Can you work these out from the model? Positions are in its coordinate system, mm. A direction names the side the tool comes from. Give positions to 0.01 mm unless a question says otherwise; leave off trailing zeros. Write each loop counter-clockwise with the first axis right and the second up, starting at its lowest first coordinate (ties: lowest second). Pieces come first, ordered by that corner, then holes. Notation, with made-up numbers: M 41,25 L 59,25 A7 cw 59,35 Z; hole C 74.5,14.5 d7. An arc over 180 degrees is marked long. Write each question's results on one line, items separated by ' | '.
from build123d import *

# Parameters (mm, degrees)
F0_R     = 1.190625
F1_DEPTH = 4.7625
F2_R     = 1.27


# Not quite as in the source:
# - a feature names something its author has since deleted; it is built from what else it names


with BuildPart() as f1:
    # F0 (on Front) → F1 (new body)
    with BuildSketch(Plane.XZ):
        with BuildLine():
            Line((0, 5.08), (5.08, 5.08))
            Line((5.08, 5.08), (5.08, 14.605))
            Line((5.08, 14.605), (5.08, 24.13))
            Line((5.08, 24.13), (0, 24.13))
            Line((0, 24.13), (0, 21.844))
            ThreePointArc((0, 21.844), (1.9756563466, 21.0256563466), (2.794, 19.05))
            ThreePointArc((2.794, 19.05), (1.9756563466, 17.0743436534), (0, 16.256))
            Line((0, 16.256), (0, 5.08))
        make_face()
        with BuildLine():
            Line((-5.08, 5.08), (0, 5.08))
            Line((0, 5.08), (0, 16.256))
            ThreePointArc((0, 16.256), (-2.794, 19.05), (0, 21.844))
            Line((0, 21.844), (0, 24.13))
            Line((0, 24.13), (-5.08, 24.13))
            Line((-5.08, 24.13), (-5.08, 5.08))
        make_face()
        Polygon((35.56, -5.08), (35.56, 5.08), (5.08, 5.08), (0, 5.08), (-5.08, 5.08), (-35.56, 5.08), (-35.56, -5.08), align=None)
        with Locations((-30.48, 0)):
            Circle(F0_R, mode=Mode.SUBTRACT)
        with Locations((30.48, 0)):
            Circle(F0_R, mode=Mode.SUBTRACT)
    extrude(amount=F1_DEPTH)

    # F2
    f2_edges = [f1.edges().sort_by_distance(p)[0] for p in [
        (-5.08, -2.38125, 24.13),
        (5.08, -2.38125, 24.13),
        (35.56, -2.38125, 5.08),
        (35.56, -2.38125, -5.08),
        (-35.56, -2.38125, -5.08),
        (-35.56, -2.38125, 5.08),
    ]]
    fillet(f2_edges, radius=F2_R)


solid = f1.part
Item 1: I want a section at C-C, the plane z = 18.25. Please give me the cut outline in (x, y), and give its area (3 significant figures).
Geometry says:
outline: M -5.08,-4.76 L -2.68,-4.76 L -2.68,0 L -5.08,0 Z; M 2.68,-4.76 L 5.08,-4.76 L 5.08,0 L 2.68,0 Z | area: 22.9 mm2
Item 2: If I drill on line 1 (Z direction, x = -30.48, y = -1.25); line 2 (X direction, y = -2.8, z = 8); line 3 (X direction, y = -0.7, z = -1), over which ranges is the centre line in solid material (lowest first)? Write a range as from..to.
Geometry says:
line 1: z = -5.08..-1.19, 1.19..5.08 | line 2: x = -5.08..5.08 | line 3: x = -35.56..-31.13, -29.83..29.83, 31.13..35.56
Item 3: I want a section at B-B, the plane y = -3.3. Please give me the cut outline in (x, z).
Geometry says:
outline: M -35.56,-3.81 A1.27 ccw -34.29,-5.08 L 34.29,-5.08 A1.27 ccw 35.56,-3.81 L 35.56,3.81 A1.27 ccw 34.29,5.08 L 5.08,5.08 L 5.08,22.86 A1.27 ccw 3.81,24.13 L -3.81,24.13 A1.27 ccw -5.08,22.86 L -5.08,5.08 L -34.29,5.08 A1.27 ccw -35.56,3.81 Z; hole C -30.48,0 d2.38; hole C 0,19.05 d5.59; hole C 30.48,0 d2.38
Item 4: I'm going to push flat-ended pins straight in: pin 1 (4 mm diameter, centred on x = 8, z = 18.5, fed in from -Y); pin 2 (1.4 mm diameter, centred on x = -15, y = -2, fed in from +Z); pin 3 (1.5 mm diameter, centred on y = -2, z = 21, fed in from -X). Where does each tip first touch, or does it pass through?
Geometry says:
pin 1: passes through | pin 2: stops at z = 5.08 | pin 3: stops at x = -5.08
Item 5: I want a section at A-A, the plane x = 30.48. Please give me the cut outline in (y, z), and give its area (3 significant figures).
Geometry says:
outline: M -4.76,-5.08 L 0,-5.08 L 0,-1.19 L -4.76,-1.19 Z; M -4.76,1.19 L 0,1.19 L 0,5.08 L -4.76,5.08 Z | area: 37.0 mm2
Item 6: I want a section at D-D, the plane z = 13.5. Please give me the cut outline in (x, y), and give its area (3 significant figures).
Geometry says:
outline: M -5.08,-4.76 L 5.08,-4.76 L 5.08,0 L -5.08,0 Z | area: 48.4 mm2
Item 7: Thinking about a two-plate mould opening in Z: for faces 4 (the face through (5.08, -2, 14)), 5 (the face through (-19, -2, 5.08)), 6 (the face through (31.58, -2.35, -0.46)), 7 (the face through (-31.67, -2.35, 0.05)), which applies, +Z half, -Z half, draft (parallel to the pull), parting line (faces both ways), or undercut?
Geometry says:
face 4: draft | face 5: +Z half | face 6: undercut | face 7: undercut
Item 8: For faces 1 (the face through (-35.56, -2, 0)), 2 (the face through (20, -2, 5.08)), 3 (the face through (-5.08, -2, 14)), which set-ups out of +Z, -Z, +X, -X, +Y, -Y let a thin tool reach every point of the face, with its end or its side?
Geometry says:
face 1: +Z, -Z, -X, +Y, -Y | face 2: +Z, +X, +Y, -Y | face 3: +Z, -X, +Y, -Y
